For this review, take the finished solid that the model builds, in its own axes (mm). A direction names the side the tool comes from. Coordinates: 2 decimals unless noted, no trailing zeros. Loops run counter-clockwise (first coordinate to the right, second up) from the corner with the lowest first, then second, coordinate; pieces in that order, holes last. Notation, with made-up numbers: M 23,61.25 L 45,61.25 A8 ccw 45,74.25 Z; hole C 8,18.25 d6. An arc over 180 degrees is marked long. Write item = value, one per line.
from build123d import *

# Parameters (mm, degrees)
SKETCH_1_W                       = 44
SKETCH_1_H                       = 36
SM_BASE_FLANGE_1_DEPTH           = 2
SM_EDGE_FLANGE_3_STRIP_W         = 9.4732
SM_EDGE_FLANGE_3_STRIP_H         = 2
SM_EDGE_FLANGE_3_STRIP_CUT_DEPTH = 36
SM_EDGE_FLANGE_3_DEPTH           = 36
SM_EDGE_FLANGE_4_STRIP_W         = 9.4732
SM_EDGE_FLANGE_4_STRIP_H         = 2
SM_EDGE_FLANGE_4_STRIP_CUT_DEPTH = 36
SM_EDGE_FLANGE_4_DEPTH           = 36
CUT_EXTRUDE_2_DEPTH              = 50
SKETCH_20_R                      = 1
CUT_EXTRUDE_3_DEPTH              = 50
FILLET_2_R                       = 2
FILLET_3_R                       = 2
FILLET_4_R                       = 2
FILLET_5_R                       = 2
FILLET_8_R                       = 2
FILLET_9_R                       = 2
FILLET_10_R                      = 2
FILLET_11_R                      = 2
SKETCH_21_R                      = 3
SKETCH_21_R_2                    = 1.5
CUT_EXTRUDE_4_DEPTH              = 2
SKETCH_22_R                      = 4
CUT_EXTRUDE_5_DEPTH              = 50


# Sheet-metal steps are written as plain solids
with BuildPart() as part:
    # Sketch 1 → 基体-法兰1 (new body)
    with BuildSketch(Plane.XY):
        with Locations((1.829071755, 6.237870574)):
            Rectangle(SKETCH_1_W, SKETCH_1_H)
    extrude(amount=-SM_BASE_FLANGE_1_DEPTH)

    # 边线-法兰3 strip (across the edge) → 边线-法兰3 strip cut (cut)
    with BuildSketch(Plane(origin=(-20.170928245, 24.237870574, 0), x_dir=(1, 0, 0), z_dir=(0, -1, 0))):
        with Locations((-2, -1)):
            Rectangle(SM_EDGE_FLANGE_3_STRIP_W, SM_EDGE_FLANGE_3_STRIP_H)
    extrude(amount=SM_EDGE_FLANGE_3_STRIP_CUT_DEPTH, mode=Mode.SUBTRACT)

    # 边线-法兰3 section (across the edge) → 边线-法兰3 (add)
    with BuildSketch(Plane(origin=(-20.170928245, 24.237870574, 0), x_dir=(1, 0, 0), z_dir=(0, -1, 0))):
        with BuildLine():
            Line((0, 0.7366), (0, 26))
            Line((0, 26), (2, 26))
            Line((2, 26), (2, 0.7366))
            ThreePointArc((2, 0.7366), (2.215745145, 0.215745145), (2.7366, 0))
            Line((2.7366, 0), (2.7366, -2))
            ThreePointArc((2.7366, -2), (0.801531583, -1.198468417), (0, 0.7366))
        make_face()
    extrude(amount=SM_EDGE_FLANGE_3_DEPTH)

    # 边线-法兰4 strip (across the edge) → 边线-法兰4 strip cut (cut)
    with BuildSketch(Plane(origin=(23.829071755, -11.762129426, 0), x_dir=(-1, 0, 0), z_dir=(0, 1, 0))):
        with Locations((-2, -1)):
            Rectangle(SM_EDGE_FLANGE_4_STRIP_W, SM_EDGE_FLANGE_4_STRIP_H)
    extrude(amount=SM_EDGE_FLANGE_4_STRIP_CUT_DEPTH, mode=Mode.SUBTRACT)

    # 边线-法兰4 section (across the edge) → 边线-法兰4 (add)
    with BuildSketch(Plane(origin=(23.829071755, -11.762129426, 0), x_dir=(-1, 0, 0), z_dir=(0, 1, 0))):
        with BuildLine():
            Line((0, 0.7366), (0, 26))
            Line((0, 26), (2, 26))
            Line((2, 26), (2, 0.7366))
            ThreePointArc((2, 0.7366), (2.215745145, 0.215745145), (2.7366, 0))
            Line((2.7366, 0), (2.7366, -2))
            ThreePointArc((2.7366, -2), (0.801531583, -1.198468417), (0, 0.7366))
        make_face()
    extrude(amount=SM_EDGE_FLANGE_4_DEPTH)

    # 草图19 → 切除-拉伸2 (cut)
    with BuildSketch(Plane.ZY.offset(20.170928245)):
        Polygon((6, 16.237870574), (26, 16.237870574), (26, 24.237870574), (0.7366, 24.237870574), align=None)
        Polygon((26, -11.762129426), (26, -3.762129426), (6, -3.762129426), (0.7366, -11.762129426), align=None)
    extrude(amount=-CUT_EXTRUDE_2_DEPTH, mode=Mode.SUBTRACT)

    # 草图20 → 切除-拉伸3 (cut)
    with BuildSketch(Plane.ZY.offset(20.170928245)):
        with Locations((23.5, 13.737870574)):
            Circle(SKETCH_20_R)
        with Locations((8.5, 13.737870574)):
            Circle(SKETCH_20_R)
        with Locations((8.5, -1.262129426)):
            Circle(SKETCH_20_R)
        with Locations((23.5, -1.262129426)):
            Circle(SKETCH_20_R)
        with Locations((9, 6.237870574)):
            Circle(SKETCH_20_R)
        with Locations((16, -0.762129426)):
            Circle(SKETCH_20_R)
        with Locations((16, 13.237870574)):
            Circle(SKETCH_20_R)
    extrude(amount=-CUT_EXTRUDE_3_DEPTH, mode=Mode.SUBTRACT)

    # 圆角2
    fillet_2_edges = [part.edges().sort_by_distance(p)[0] for p in [
        (-19.170928245, -3.762129426, 26),
    ]]
    fillet(fillet_2_edges, radius=FILLET_2_R)

    # 圆角3
    fillet_3_edges = [part.edges().sort_by_distance(p)[0] for p in [
        (-19.170928245, 16.237870574, 26),
    ]]
    fillet(fillet_3_edges, radius=FILLET_3_R)

    # 圆角4
    fillet_4_edges = [part.edges().sort_by_distance(p)[0] for p in [
        (22.829071755, 16.237870574, 26),
    ]]
    fillet(fillet_4_edges, radius=FILLET_4_R)

    # 圆角5
    fillet_5_edges = [part.edges().sort_by_distance(p)[0] for p in [
        (22.829071755, -3.762129426, 26),
    ]]
    fillet(fillet_5_edges, radius=FILLET_5_R)

    # 圆角8
    fillet_8_edges = [part.edges().sort_by_distance(p)[0] for p in [
        (22.829071755, -3.762129426, 6),
    ]]
    fillet(fillet_8_edges, radius=FILLET_8_R)

    # 圆角9
    fillet_9_edges = [part.edges().sort_by_distance(p)[0] for p in [
        (22.829071755, 16.237870574, 6),
    ]]
    fillet(fillet_9_edges, radius=FILLET_9_R)

    # 圆角10
    fillet_10_edges = [part.edges().sort_by_distance(p)[0] for p in [
        (-19.170928245, 16.237870574, 6),
    ]]
    fillet(fillet_10_edges, radius=FILLET_10_R)

    # 圆角11
    fillet_11_edges = [part.edges().sort_by_distance(p)[0] for p in [
        (-19.170928245, -3.762129426, 6),
    ]]
    fillet(fillet_11_edges, radius=FILLET_11_R)

    # 草图21 → 切除-拉伸4 (cut)
    with BuildSketch(Plane(origin=(0, 0, -2), x_dir=(-1, 0, 0), z_dir=(0, 0, -1))):
        with Locations((-1.829071755, 6.237870574)):
            Circle(SKETCH_21_R)
        with Locations((3.120675713, 11.187618042)):
            Circle(SKETCH_21_R_2)
        with Locations(Location((-6.778819223, 11.187618042, 0), (0, 0, 180))):
            Circle(SKETCH_21_R_2)
        with Locations((-6.778819223, 1.288123106)):
            Circle(SKETCH_21_R_2)
        with Locations(Location((3.120675713, 1.288123106, 0), (0, 0, 180))):
            Circle(SKETCH_21_R_2)
    extrude(amount=-CUT_EXTRUDE_4_DEPTH, mode=Mode.SUBTRACT)

    # 草图22 → 切除-拉伸5 (cut)
    with BuildSketch(Plane.ZY.offset(20.170928245)):
        with Locations((16, 6.237870574)):
            Circle(SKETCH_22_R)
    extrude(amount=-CUT_EXTRUDE_5_DEPTH, mode=Mode.SUBTRACT)


solid = part.part
Q1. For line 1 along Y through (x, z) = (-19.4, 23.5); line 2 along Y through (x, z) = (-18.85, 16); line 3 along X through (y, z) = (-4, 1.5), list the stretches that pass through material, from the lowest coordinate up.
Solved:
line_1 = -3.76 to -2.26, -0.26 to 12.74, 14.74 to 16.24
line_2 = -3.76 to -1.76, 0.24 to 2.24, 10.24 to 12.24, 14.24 to 16.24
line_3 = -20.17 to -18.17, 21.83 to 23.83
Q2. Machinability: for faces 1 (the face through (22.82, -0.59, 22.76)), 2 (the face through (-18.171, 6, 11)), 3 (the face through (23, 16.238, 15)), 4 (the face through (23, -3.762, 16)), which of the approach directions +Z, -Z, +X, -X, +Y, -Y give a long, thin tool a straight path to every point of the face, cutting with its end or side? Answer none if there is none.
Solved:
face_1 = +X, -X
face_2 = +Z, +Y, -Y
face_3 = +Z, +X, -X, +Y
face_4 = +Z, +X, -X, -Y
Q3. Add section D-D (x = -2.5). Write out the cut boundary in (y, z), and give its area (3 significant figures).
Solved:
outline = M -11.76,-2 L -0.08,-2 L -0.08,0 L -11.76,0 Z; M 2.65,-2 L 9.82,-2 L 9.82,0 L 2.65,0 Z; M 12.55,-2 L 24.24,-2 L 24.24,0 L 12.55,0 Z
area = 61.1 mm²
Q4. Add section A-A (z = 16). State how many separate pieces and enclosed holes the cut face has, and give its area (3 significant figures).
Solved:
separate_pieces = 8
enclosed_holes = 0
area = 32.0 mm²
Q5. Add section C-C (z = 21). Write out the cut boundary in (x, y), and give its area (3 significant figures).
Solved:
outline = M -20.17,-3.76 L -18.17,-3.76 L -18.17,16.24 L -20.17,16.24 Z; M 21.83,-3.76 L 23.83,-3.76 L 23.83,16.24 L 21.83,16.24 Z
area = 80.0 mm²
Q6. For pin 1 Ø1.6 at (x, z) = (23, 17) entering from +Y; pin 2 Ø1 at (x, z) = (-19, 15.5) entering from -Y; pin 3 Ø3 at (x, y) = (11, 20.5) entering from +Z, all flat-tipped, find the tip position at first contact; note any pin that passes through.
Solved:
pin_1 = 16.24
pin_2 = -3.76
pin_3 = 0
Q7. Add section B-B (x = 2). Write out the cut boundary in (y, z), and give its area (3 significant figures).
Solved:
outline = M -11.76,-2 L 3.24,-2 L 3.24,0 L -11.76,0 Z; M 9.23,-2 L 24.24,-2 L 24.24,0 L 9.23,0 Z
area = 60.0 mm²
Q8. Draft analysis for pull direction X (two halves, no side actions). For faces 5 (the face through (8.21, 10.74, -1.01)), 6 (the face through (-19, -3.762, 16)), 7 (the face through (23.829, 6, 10.4)), state which applies: +X half, -X half, draft (parallel to the pull), parting line (faces both ways), or undercut.
Solved:
face_5 = undercut
face_6 = draft
face_7 = +X half
